The figure shows three views and two pictorial views of one solid part (mm, origin at its lowest corner). Answer the questions. Coordinates: 2 decimals unless noted, no trailing zeros. Order: outer loops, then holes, each group sorted by start corner. A loop starts at its lowest first (then second) coordinate and runs counter-clockwise, first axis right, second up. Notation, with made-up numbers: (75, -33.5) -> (127, -33.5) arc R31 ccw to (127, -8.5) -> close; hole circle Ø5 at (-34, 75.5). An arc over 180 degrees is marked (long way). Return JSON: item names as keys, results as strings.
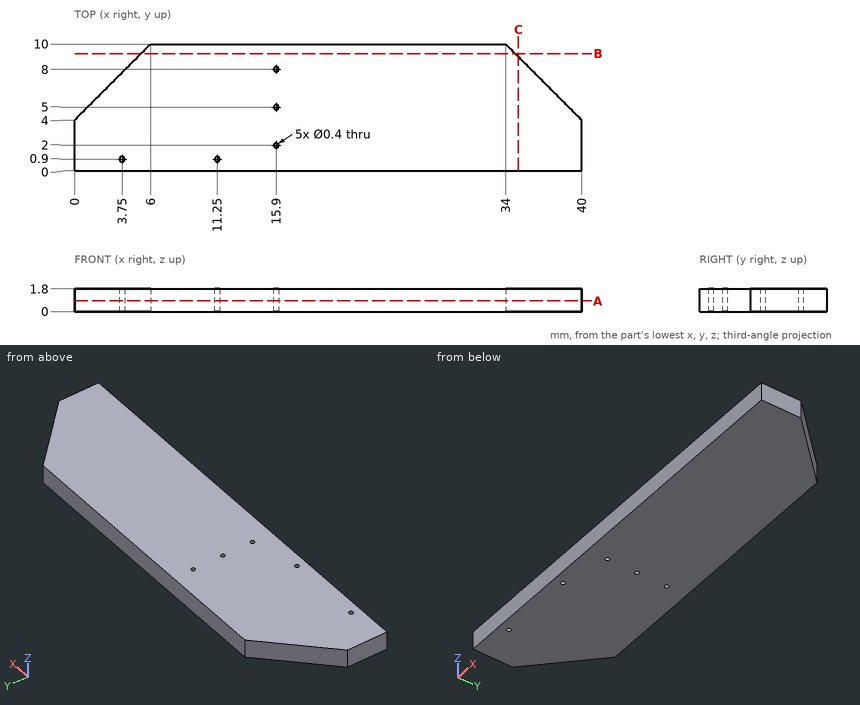
1. The part is cut by section C-C on x = 35. Give the vertices of the cut face in (y, z), and give its area (3 significant figures).
Answer block:
{"outline": "(0, 0) -> (9, 0) -> (9, 1.8) -> (0, 1.8) -> close", "area": "16.2 mm2"}
2. Consider line 1 (Y direction, x = 15.9, z = 0.65); line 2 (X direction, y = 8, z = 1.4); line 3 (X direction, y = 5, z = 1.3). Determine where each line is inside the solid, lowest interval first. Write a range as from..to.
Answer block:
{"line 1": "y = 0..1.8, 2.2..4.8, 5.2..7.8, 8.2..10", "line 2": "x = 4..15.7, 16.1..36", "line 3": "x = 1..15.7, 16.1..39"}
3. The part is cut by section A-A on z = 0.85. Give the vertices of the cut face in (x, y), and give its area (3 significant figures).
Answer block:
{"outline": "(0, 0) -> (40, 0) -> (40, 4) -> (34, 10) -> (6, 10) -> (0, 4) -> close; hole circle Ø0.4 at (3.75, 0.9); hole circle Ø0.4 at (11.25, 0.9); hole circle Ø0.4 at (15.9, 2); hole circle Ø0.4 at (15.9, 5); hole circle Ø0.4 at (15.9, 8)", "area": "363 mm2"}
4. The part is cut by section B-B on y = 9.25. Give the vertices of the cut face in (x, z).
Answer block:
{"outline": "(5.25, 0) -> (34.75, 0) -> (34.75, 1.8) -> (5.25, 1.8) -> close"}
